Could you check a few things on this drawing? It's one solid part, dimensions in mm from its lowest x, y, z. A direction names the side the tool comes from. Round coordinates to 2 decimals unless told otherwise and drop trailing zeros. Write each loop counter-clockwise with the first axis right and the second up, starting at its lowest first coordinate (ties: lowest second). Pieces come first, ordered by that corner, then holes. Notation, with made-up numbers: (-33.5, 72) - (18.5, 72) arc R23 ccw to (18.5, 95) - close; hole circle Ø7 at (-26.5, 34.5). An arc over 180 degrees is marked (long way). Write item = value, one per line. Start each with the question number.
Item 1: If we section it at B-B (y = 144): Please give me the cut outline in (x, z).
Item 2: If we section it at A-A (z = 60.5): Please give me the cut outline in (x, y), and give its area (3 significant figures).
Item 3: If I drill on line 1 along X through (y, z) = (118, 48); line 2 along X through (y, z) = (21, 62), over which ranges is the centre line in solid material (lowest first)? Write a range as [from, to].
Item 4: Thinking about a two-plate mould opening in Y: for the marked faces 1, 2, 3 and 4, which applies, pulls with the +Y half, pulls with the -Y half, needs draft (parallel to the pull), parting line crosses it, or undercut?
Item 5: Which directions (+Z, -Z, +X, -X, +Y, -Y) give clear straight access to the entire face, cutting with the end or side of a thin tool? Please do the marked faces 5 and 6.
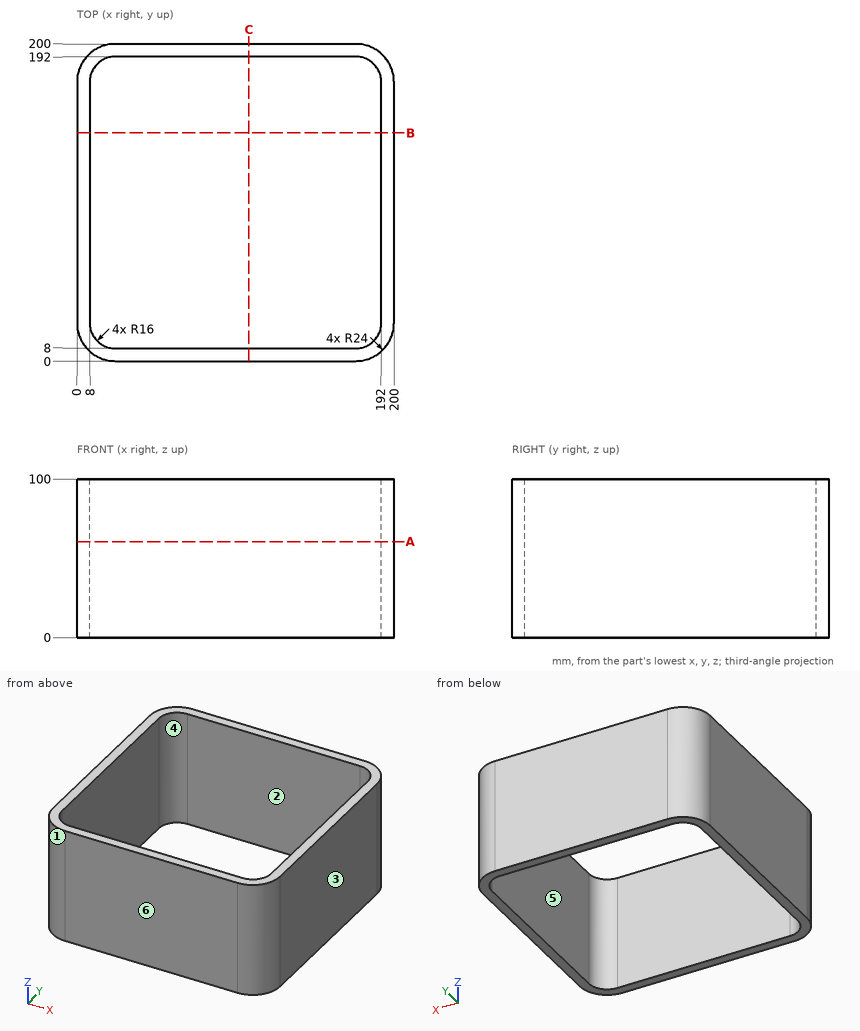
Reply:
q1.outline = (0, 0) - (8, 0) - (8, 100) - (0, 100) - close; (192, 0) - (200, 0) - (200, 100) - (192, 100) - close
q2.outline = (0, 24) arc R24 ccw to (24, 0) - (176, 0) arc R24 ccw to (200, 24) - (200, 176) arc R24 ccw to (176, 200) - (24, 200) arc R24 ccw to (0, 176) - close; hole (8, 24) arc R16 ccw to (24, 8) - (176, 8) arc R16 ccw to (192, 24) - (192, 176) arc R16 ccw to (176, 192) - (24, 192) arc R16 ccw to (8, 176) - close
q2.area = 5,870 mm2
q3.line_1 = [0, 8], [192, 200]
q3.line_2 = [0.19, 8.28], [191.72, 199.81]
q4.face_1 = pulls with the -Y half
q4.face_2 = undercut
q4.face_3 = needs draft
q4.face_4 = undercut
q5.face_5 = +Z, -Z
q5.face_6 = +Z, -Z, +X, -X, -Y
